CAD build for the part. Positions are in the model's coordinates, mm. A direction names the side the tool comes from. Give positions to 0.01 mm unless a question says otherwise; leave off trailing zeros. Loops run counter-clockwise (first coordinate to the right, second up) from the corner with the lowest first, then second, coordinate; pieces in that order, holes last.
```python
from build123d import *

# Parameters (mm, degrees)
SKIZZE1_R                       = 2.795
AUFSATZ_LINEAR_AUSTRAGEN1_DEPTH = 94.27
AUFSATZ_LINEAR_AUSTRAGEN2_DEPTH = 62.74
SCHNITT_LINEAR_START            = 94.27
SCHNITT_LINEAR_AUSTRAGEN1_DEPTH = 10


with BuildPart() as part:
    # Skizze1 → Aufsatz-Linear austragen1 (new body)
    with BuildSketch(Plane(origin=(0, 0, 0), x_dir=(0, 0, -1), z_dir=(1, 0, 0))):
        Circle(SKIZZE1_R)
    extrude(amount=AUFSATZ_LINEAR_AUSTRAGEN1_DEPTH)

    # Skizze2 → Aufsatz-Linear austragen2 (add)
    with BuildSketch(Plane(origin=(11, 0, 0), x_dir=(0, 0, -1), z_dir=(1, 0, 0))):
        Polygon((1.613694002, 2.795), (-1.613694002, 2.795), (-3.227388005, 0), (-1.613694002, -2.795), (1.613694002, -2.795), (3.227388005, 0), align=None)
    extrude(amount=AUFSATZ_LINEAR_AUSTRAGEN2_DEPTH)

    # Skizze3 → Schnitt-Linear austragen1 (cut)
    with BuildSketch(Plane(origin=(0, 0, 0), x_dir=(0, 0, -1), z_dir=(1, 0, 0)).offset(SCHNITT_LINEAR_START)):
        with BuildLine():
            Line((1.779887637, 2.155), (-1.779887637, 2.155))
            ThreePointArc((-1.779887637, 2.155), (0, 2.795), (1.779887637, 2.155))
        make_face()
    extrude(amount=-SCHNITT_LINEAR_AUSTRAGEN1_DEPTH, mode=Mode.SUBTRACT)


solid = part.part
```
1. Saw through at A-A, the plane x = 76. List the corners of the cut face in (y, z) (3 decimals).
Responses:
outline: circle Ø5.59 at (0, 0)
2. Probe line 1 along X through (y, z) = (2.5, -1.5); line 2 along Z through (x, y) = (10.5, 0.3); line 3 along Z through (x, y) = (39, 2.5). List the from-to ranges inside material, lowest first.
Responses:
line 1: x = 11 to 73.74
line 2: z = -2.78 to 2.78
line 3: z = -1.78 to 1.78
3. Saw through at B-B, the plane x = 65. List the corners of the cut face in (y, z) (3 decimals).
Responses:
outline: (-2.795, -1.614) - (0, -3.227) - (2.795, -1.614) - (2.795, 1.614) - (0, 3.227) - (-2.795, 1.614) - close
4. Drop flat-ended pins along their axis: pin 1 (0.9 mm diameter, centred on y = 0.5, z = 3, fed in from +X); pin 2 (1.5 mm diameter, centred on x = 15.5, z = -2.5, fed in from -Y); pin 3 (0.5 mm diameter, centred on y = 2.5, z = 0, fed in from +X); pin 4 (2 mm diameter, centred on x = 41.5, y = -1.5, fed in from -Z). Give the stop position or say it passes through.
Responses:
pin 1: stops at x = 94.27
pin 2: stops at y = -2.56
pin 3: stops at x = 84.27
pin 4: stops at z = -2.94
5. Tool access for faces 1 (the face through (5.423, 0.84, -2.666)), 2 (the face through (89, 2.155, 0)), 3 (the face through (94.27, 0, 0)), 4 (the face through (83.861, -2.729, 0.606)): list every direction of +Z, -Z, +X, -X, +Y, -Y with a clear straight run to the whole face (end or side of a thin tool).
Responses:
face 1: -X
face 2: +Z, -Z, +X, +Y
face 3: +Z, -Z, +X, +Y, -Y
face 4: +X
